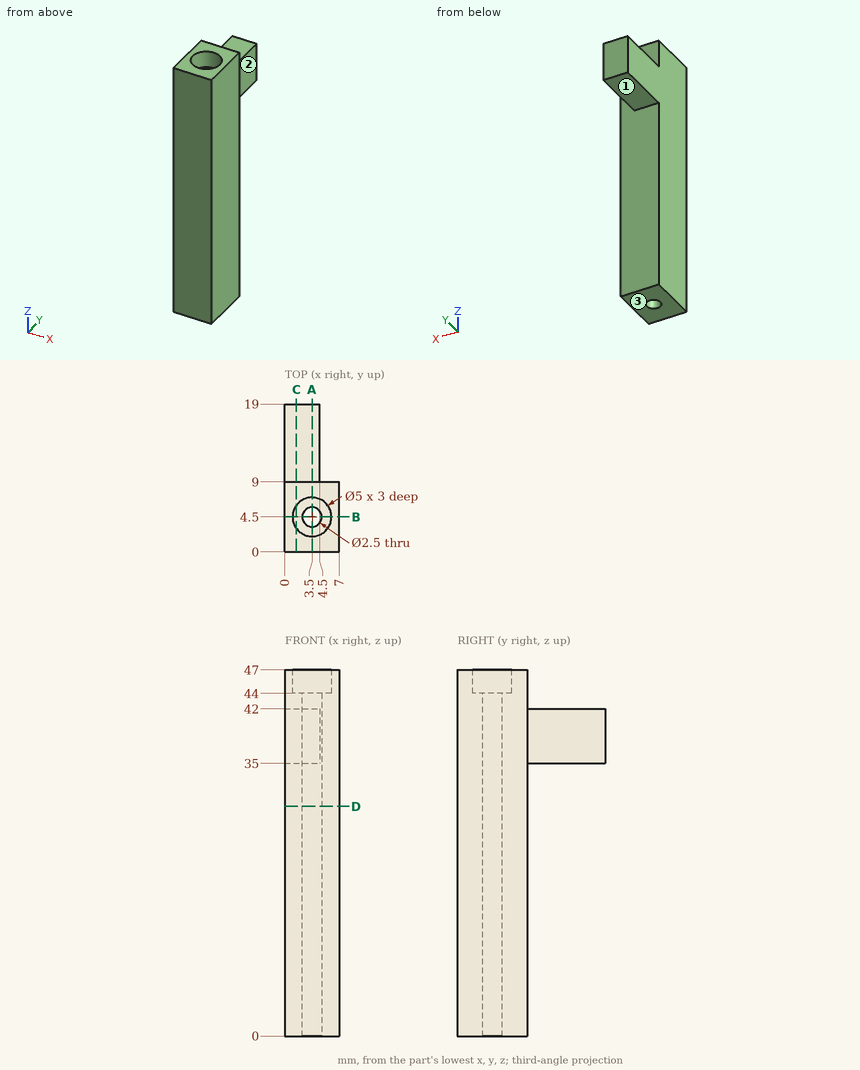
Could you check a few things on this drawing? It's one solid part, dimensions in mm from its lowest x, y, z. A direction names the side the tool comes from. Coordinates: 2 decimals unless noted, no trailing zeros. Write each loop counter-clockwise with the first axis right and the second up, starting at its lowest first coordinate (ties: lowest second). Pieces come first, ordered by that corner, then holes. Notation, with made-up numbers: (-19.75, 43.25) - (17.25, 43.25) arc R10 ccw to (17.25, 48.25) - close; hole circle Ø11 at (75, 62.5). An arc over 180 degrees is marked (long way). Write item = value, one per line.
1) Suppose I cut it at A-A on x = 3.5. Please give me the cut outline in (y, z).
Result set:
outline = (0, 0) - (3.25, 0) - (3.25, 44) - (2, 44) - (2, 47) - (0, 47) - close; (5.75, 0) - (9, 0) - (9, 35) - (19, 35) - (19, 42) - (9, 42) - (9, 47) - (7, 47) - (7, 44) - (5.75, 44) - close
2) Suppose I cut it at D-D on z = 29.5. Please give me the cut outline in (x, y), plus the area to 3 significant figures.
Result set:
outline = (0, 0) - (7, 0) - (7, 9) - (0, 9) - close; hole circle Ø2.5 at (3.5, 4.5)
area = 58.1 mm2
3) Suppose I cut it at B-B on y = 4.5. Please give me the cut outline in (x, z), plus the area to 3 significant figures.
Result set:
outline = (0, 0) - (2.25, 0) - (2.25, 44) - (1, 44) - (1, 47) - (0, 47) - close; (4.75, 0) - (7, 0) - (7, 47) - (6, 47) - (6, 44) - (4.75, 44) - close
area = 204 mm2
4) Will these pins go through, and if not, where does the flat tip stop? pin 1 Ø2 at (x, z) = (2, 13.5) entering from +Y; pin 2 Ø2 at (x, y) = (1.5, 16) entering from +Z; pin 3 Ø2 at (x, y) = (2, 3.5) entering from +Z; pin 4 Ø8 at (y, z) = (13.5, 24.5) entering from +X.
Result set:
pin_1 = 9
pin_2 = 42
pin_3 = 47
pin_4 = through
5) For the marked faces 1, 2 and 3, which set-ups out of +Z, -Z, +X, -X, +Y, -Y let a thin tool reach every point of the face, with its end or its side?
Result set:
face_1 = -Z, +X, -X, +Y
face_2 = +Z, -Z, +X, +Y
face_3 = -Z, +X, -X, +Y, -Y
6) Suppose I cut it at C-C on x = 1.5. Please give me the cut outline in (y, z), plus the area to 3 significant figures.
Result set:
outline = (0, 0) - (9, 0) - (9, 35) - (19, 35) - (19, 42) - (9, 42) - (9, 47) - (6, 47) - (6, 44) - (3, 44) - (3, 47) - (0, 47) - close
area = 484 mm2
7) Please list where these lines run through material, in increasing order: line 1 (Y direction, x = 3.5, z = 15.5); line 2 (Z direction, x = 1.75, y = 14.75); line 3 (Y direction, x = 3.5, z = 45). Write a range as [from, to].
Result set:
line_1 = [0, 3.25], [5.75, 9]
line_2 = [35, 42]
line_3 = [0, 2], [7, 9]
